Geometry check sheet. Reference: the model listing, model coordinates, mm. Round coordinates to 2 decimals unless told otherwise and drop trailing zeros. Order: outer loops, then holes, each group sorted by start corner. A loop starts at its lowest first (then second) coordinate and runs counter-clockwise, first axis right, second up. Notation, with made-up numbers: (74.5, 59.25) -> (123.5, 59.25) arc R27 cw to (123.5, 80.25) -> close; hole circle Ø4 at (-36, -36.5). An arc over 180 degrees is marked (long way). Answer as a JSON object with one key per item and string values. Group by question number.
from build123d import *

# Parameters (mm, degrees)
SKETCH_2_R      = 3
EXTRUDE_2_DEPTH = 1.6
FILLET_START    = -1
FILLET_1_DEPTH  = 4


with BuildPart() as part:
    # Sketch 2 → Extrude 2 (new body)
    with BuildSketch(Plane.XY):
        with BuildLine():
            ThreePointArc((28.284271247, 28.284271247), (-15.307337295, 36.9551813), (-40, 0))
            Line((-40, 0), (-40, -70))
            Line((-40, -70), (70, -70))
            Line((70, -70), (70, -13.431457505))
            Line((70, -13.431457505), (28.284271247, 28.284271247))
        make_face()
        with Locations((0, -19.5)):
            Circle(SKETCH_2_R, mode=Mode.SUBTRACT)
        with BuildLine():
            Line((25.4460213, -9.75), (9.75, -9.75))
            Line((9.75, -9.75), (6.99553429, -9.75))
            ThreePointArc((6.99553429, -9.75), (0, -12), (-6.99553429, -9.75))
            Line((-6.99553429, -9.75), (-25.4460213, -9.75))
            ThreePointArc((-25.4460213, -9.75), (-27.25, 0), (-25.4460213, 9.75))
            Line((-25.4460213, 9.75), (-6.99553429, 9.75))
            ThreePointArc((-6.99553429, 9.75), (0, 12), (6.99553429, 9.75))
            Line((6.99553429, 9.75), (25.4460213, 9.75))
            ThreePointArc((25.4460213, 9.75), (27.25, 0), (25.4460213, -9.75))
        make_face(mode=Mode.SUBTRACT)
        with Locations((0, 19.5)):
            Circle(SKETCH_2_R, mode=Mode.SUBTRACT)
    extrude(amount=EXTRUDE_2_DEPTH)

    # Fillet 1: read off the stored shape, not the designer's step
    # Fillet 1 outline → Fillet 1 (cut)
    with BuildSketch(Plane.XY.offset(FILLET_START)):
        with BuildLine():
            Line((70, -13.431457505), (67.071067812, -10.502525317))
            add(Edge.make_bspline(
                [(67.071067812, -10.502525317), (70, -13.431457505), (70, -17.573593129)],
                knots=[0, 0, 0, 1, 1, 1], degree=2, weights=[1, 0.923879533, 1]))
            Line((70, -17.573593129), (70, -13.431457505))
        make_face()
    extrude(amount=FILLET_1_DEPTH, mode=Mode.SUBTRACT)


solid = part.part
Item 1: Sectioned sample at A-A, the plane y = -19.5. Enter the section's corners in (x, z).
Item 2: Depth check by flat-ended pin: pin 1 Ø0.5 at (x, z) = (17, 1) entering from +Y; pin 2 Ø3.5 at (x, y) = (0, -19.5) entering from -Z; pin 3 Ø0.5 at (x, z) = (-18.5, 1) entering from +Y. Enter the tip coordinate at first touch or a pass-through.
Item 3: Mould release check, pull along X, two halves, no side actions. Record for faces 1 (the cylindrical face through (-14.7, 37.2, 0.8)), 2 (the flat face through (14, -26, 0)), 3 (the cylindrical face through (-0.65, 16.57, 0.79)): pulls with the +X half, pulls with the -X half, needs draft (parallel to the pull), parting line crosses it, or undercut.
Item 4: Sectioned sample at B-B, the plane x = 0. Enter the section's corners in (y, z).
Item 5: Sectioned sample at D-D, the plane z = 0.85. Count the separate pieces of the cut face and the enclosed holes in it, then the cut area to 3 significant figures.
Item 6: Sectioned sample at C-C, the plane x = -20. Enter the section's corners in (y, z).
Item 7: Thickness scan on L1, parallel to Y at x = 0, z = 0.55; L2, parallel to Y at x = -18.5, z = 1.55; L3, parallel to X at y = 19, z = 0.55. Record the ranges inside material, lowest first.
Result:
{
 "1": {"outline": "(-40, 0) -> (-3, 0) -> (-3, 1.6) -> (-40, 1.6) -> close; (3, 0) -> (70, 0) -> (70, 1.6) -> (3, 1.6) -> close"},
 "2": {"pin 1": "stops at y = 36.32", "pin 2": "passes through", "pin 3": "stops at y = 35.59"},
 "3": {"face 1": "parting line crosses it", "face 2": "needs draft", "face 3": "undercut"},
 "4": {"outline": "(-70, 0) -> (-22.5, 0) -> (-22.5, 1.6) -> (-70, 1.6) -> close; (-16.5, 0) -> (-12, 0) -> (-12, 1.6) -> (-16.5, 1.6) -> close; (12, 0) -> (16.5, 0) -> (16.5, 1.6) -> (12, 1.6) -> close; (22.5, 0) -> (40, 0) -> (40, 1.6) -> (22.5, 1.6) -> close"},
 "5": {"separate pieces": "1", "enclosed holes": "3", "area": "9,150 mm2"},
 "6": {"outline": "(-70, 0) -> (-9.75, 0) -> (-9.75, 1.6) -> (-70, 1.6) -> close; (9.75, 0) -> (34.64, 0) -> (34.64, 1.6) -> (9.75, 1.6) -> close"},
 "7": {"L1": "y = -70 to -22.5, -16.5 to -12, 12 to 16.5, 22.5 to 40", "L2": "y = -70 to -9.75, 9.75 to 35.46", "L3": "x = -35.2 to -2.96, 2.96 to 37.57"}
}
